from build123d import *

# Parameters (mm, degrees)
SKETCH2_W           = 304.8
SKETCH2_H           = 152.4
BOSS_EXTRUDE1_DEPTH = 152.4
SHELL1_T            = -3.175
SKETCH3_W           = 12.7
SKETCH3_H           = 6.35
CUT_EXTRUDE1_DEPTH  = 374.3022368


with BuildPart() as part:
    # Sketch2 → Boss-Extrude1 (new body)
    with BuildSketch(Plane.XY):
        with Locations((152.4, 76.2)):
            Rectangle(SKETCH2_W, SKETCH2_H)
    extrude(amount=BOSS_EXTRUDE1_DEPTH)

    # Shell1
    shell1_openings = [part.faces().sort_by_distance(p)[0] for p in [
        (152.4, 76.2, 152.4),
    ]]
    offset(amount=SHELL1_T, openings=shell1_openings, kind=Kind.INTERSECTION)

    # Sketch3 → Cut-Extrude1 (cut, through all)
    with BuildSketch(Plane.XZ):
        with Locations((152.4, 66.929)):
            Rectangle(SKETCH3_W, SKETCH3_H)
    extrude(amount=-CUT_EXTRUDE1_DEPTH, mode=Mode.SUBTRACT)


solid = part.part
The listing builds one solid part. Answer for the finished solid, in the listing's coordinates (mm). A direction names the side the tool comes from. Coordinates: 2 decimals unless noted, no trailing zeros. Order: outer loops, then holes, each group sorted by start corner. A loop starts at its lowest first (then second) coordinate and runs counter-clockwise, first axis right, second up. Notation, with made-up numbers: M 53.25,-29 L 57.25,-29 A34 cw 57.25,8 Z; hole C 78.5,89 d4. An arc over 180 degrees is marked long. Use CSV: the item, a comma, the result in double quotes.
Q1. Given pin 1 Ø8 at (x, y) = (106, 77) entering from +Z (3 decimals), flat-ended and moving along its own axis, determine where the tip first touches the part or whether it passes through.
Here are the results:
pin 1,"z = 3.175"
Q2. Straight lines are drawn through the part: L1, parallel to X at y = 7, z = 131 (3 decimals); L2, parallel to Y at x = 203.5, z = 140 (3 decimals); L3, parallel to Z at x = 222.5, y = 104 (3 decimals). For each, find the intervals that lie inside material, in ascending order.
Here are the results:
L1,"0 to 3.175, 301.625 to 304.8"
L2,"0 to 3.175, 149.225 to 152.4"
L3,"0 to 3.175"
Q3. Determine the mould class of faces 1 (the flat face through (301.625, 75, 77)), 2 (the flat face through (150, 152.4, 75)), 3 (the flat face through (0, 75, 75)) for opening direction X: pulls with the +X half, pulls with the -X half, needs draft (parallel to the pull), parting line crosses it, or undercut.
Here are the results:
face 1,"undercut"
face 2,"needs draft"
face 3,"pulls with the -X half"
Q4. Section A-A (z = 101.5) is taken. Determine the outline of the cut face in (x, y) (3 decimals).
Here are the results:
outline,"M 0,0 L 304.8,0 L 304.8,152.4 L 0,152.4 Z; hole M 3.175,3.175 L 301.625,3.175 L 301.625,149.225 L 3.175,149.225 Z"
Q5. Section C-C (y = 76) is taken. Determine the outline of the cut face in (x, z) (3 decimals).
Here are the results:
outline,"M 0,0 L 304.8,0 L 304.8,152.4 L 301.625,152.4 L 301.625,3.175 L 3.175,3.175 L 3.175,152.4 L 0,152.4 Z"
Q6. A tool of negligible diameter and unlimited length cuts with its end or side. For faces 4 (the flat face through (150, 3.175, 77)), 5 (the flat face through (304.8, 75, 75)), from which of +Z, -Z, +X, -X, +Y, -Y can it reach the whole face along a straight path? Write none if from no direction.
Here are the results:
face 4,"+Z"
face 5,"+Z, -Z, +X, +Y, -Y"
Q7. Section B-B (x = 138.5) is taken. Determine the outline of the cut face in (y, z) (3 decimals).
Here are the results:
outline,"M 0,0 L 152.4,0 L 152.4,152.4 L 149.225,152.4 L 149.225,3.175 L 3.175,3.175 L 3.175,152.4 L 0,152.4 Z"
